Autodesk Fusion 360 part; units mm, degrees
sketch "Sketch1" plane through (0, 0, 0) normal (0, 0, 1) x (1, 0, 0)
  line L0 (-19.8608, 0) -> (46.1392, 0) construction
  line L1 (-17, -9.25) -> (-10, -9.25)
  line L2 (-10, -9.25) -> (-10, -10)
  line L3 (-10, -10) -> (30.5, -10)
  line L4 (30.5, -10) -> (30.5, -9.25)
  line L5 (30.5, -9.25) -> (37.5, -9.25)
  line L6 (37.5, -9.25) -> (37.5, 0)
  circle A0 centre (-13, -4.5) radius 2.25
  line L7 (-17, -9.25) -> (-17, 0)
  circle A1 centre (34.5, -4.5) radius 2.25
  line L8 (30.5, 10) -> (30.5, 9.25)
  line L9 (-10, 9.25) -> (-10, 10)
  line L10 (-17, 9.25) -> (-17, 0)
  line L11 (37.5, 9.25) -> (37.5, 0)
  line L12 (30.5, 9.25) -> (37.5, 9.25)
  circle A2 centre (-13, 4.5) radius 2.25
  line L13 (-10, 10) -> (30.5, 10)
  line L14 (-17, 9.25) -> (-10, 9.25)
  circle A3 centre (34.5, 4.5) radius 2.25
  point P0 (46.1392, 0)
  point P1 (-19.8608, 0)
  dimension "d1" = 4.5
  dimension "d2" = 10
  dimension "d3" = 4.5
  dimension "d4" = 47.5
  dimension "d5" = 7
  dimension "d6" = 7
  dimension "d7" = 4
  dimension "d8" = 4
  dimension "d9" = 4.5
  dimension "d10" = 4.5
  dimension "d11" = 10
  dimension "d12" = 10
  dimension "d13" = 9.25
  dimension "d14" = 9.25
extrude "Extrude1" add sketch "Sketch1" along normal blind 13
sketch "Sketch3" plane through (0, -9.25, 0) normal (0, -1, 0) x (1, 0, 0)
  line L0 (30.5, 0) -> (37.5, 0)
  line L1 (37.5, 0) -> (37.5, 13)
  line L2 (37.5, 13) -> (30.5, 13)
  line L3 (30.5, 13) -> (30.5, 0)
  line L4 (37.5, 0) -> (30.5, 0)
  line L5 (30.5, 0) -> (30.5, 3)
  line L6 (30.5, 3) -> (37.5, 3)
  line L7 (37.5, 3) -> (37.5, 0)
  line L8 (-10, 0) -> (-17, 0)
  line L9 (-17, 0) -> (-17, 3)
  line L10 (-17, 3) -> (-10, 3)
  line L11 (-10, 3) -> (-10, 0)
  dimension "d21" = 3
  dimension "d22" = 3
extrude "Extrude3" cut sketch "Sketch3" against normal blind 26 contours L1 L2 L3 L6
sketch "Sketch4" plane through (0, -9.25, 0) normal (0, -1, 0) x (1, 0, 0)
  line L0 (-17, 0) -> (-10, 0)
  line L1 (-10, 0) -> (-10, 13)
  line L2 (-10, 13) -> (-17, 13)
  line L3 (-17, 13) -> (-17, 0)
  line L4 (-17, 0) -> (-10, 0)
  line L5 (-10, 0) -> (-10, 3)
  line L6 (-10, 3) -> (-17, 3)
  line L7 (-17, 3) -> (-17, 0)
  dimension "d25" = 3
extrude "Extrude4" cut sketch "Sketch4" against normal blind 22 contours L1 L2 L3 L6
sketch "Sketch5" plane through (0, 0, 13) normal (0, 0, 1) x (-1, 0, 0)
  line L0 (10, -10) -> (10, 10)
  line L1 (10, 10) -> (-30.5, 10)
  line L2 (-30.5, 10) -> (-30.5, -10)
  line L3 (-30.5, -10) -> (10, -10)
  circle A0 centre (0, 0) radius 3
  dimension "d28" = 6
extrude "Extrude5" cut sketch "Sketch5" against normal blind 21 contours A0
sketch "Sketch6" plane through (0, 0, 0) normal (0, 0, -1) x (-1, 0, 0)
  circle A0 centre (0, 0) radius 3
  line L0 (10, -10) -> (10, 10)
  line L1 (10, 10) -> (-33, 10)
  line L2 (-33, 10) -> (-33, -10)
  line L3 (-33, -10) -> (10, -10)
  circle A1 centre (-11, 0) radius 0.75
  circle A2 centre (-20.5, 0) radius 0.75
  circle A3 centre (0, 0) radius 3
  circle A4 centre (-34.5, 4.5) radius 2.25
  circle A5 centre (13, -4.5) radius 2.25
  circle A6 centre (-34.5, -4.5) radius 2.25
  circle A7 centre (13, 4.5) radius 2.25
  line L4 (10, -9.25) -> (17, -9.25)
  line L5 (17, -9.25) -> (17, 9.25)
  line L6 (17, 9.25) -> (10, 9.25)
  line L7 (10, 9.25) -> (10, 10)
  line L8 (10, 10) -> (-30.5, 10)
  line L9 (-30.5, 10) -> (-30.5, 9.25)
  line L10 (-30.5, 9.25) -> (-37.5, 9.25)
  line L11 (-37.5, 9.25) -> (-37.5, -9.25)
  line L12 (-37.5, -9.25) -> (-30.5, -9.25)
  line L13 (-30.5, -9.25) -> (-30.5, -10)
  line L14 (-30.5, -10) -> (10, -10)
  line L15 (10, -10) -> (10, -9.25)
  dimension "d31" = 1.5
  dimension "d32" = 1.5
  dimension "d33" = 11
  dimension "d34" = 9.5
extrude "Extrude6" cut sketch "Sketch6" against normal blind 12 contours A1 | A2
sketch "Sketch7" plane through (0, 0, 0) normal (0, 0, -1) x (1, 0, 0)
  circle A0 centre (11, 0) radius 0.75
  circle A1 centre (20.5, 0) radius 0.75
  circle A2 centre (0, 0) radius 3
  circle A3 centre (34.5, -4.5) radius 2.25
  circle A4 centre (-13, 4.5) radius 2.25
  circle A5 centre (34.5, 4.5) radius 2.25
  circle A6 centre (-13, -4.5) radius 2.25
  line L0 (-10, 9.25) -> (-17, 9.25)
  line L1 (-17, 9.25) -> (-17, -9.25)
  line L2 (-17, -9.25) -> (-10, -9.25)
  line L3 (-10, -9.25) -> (-10, -10)
  line L4 (-10, -10) -> (30.5, -10)
  line L5 (30.5, -10) -> (30.5, -9.25)
  line L6 (30.5, -9.25) -> (37.5, -9.25)
  line L7 (37.5, -9.25) -> (37.5, 9.25)
  line L8 (37.5, 9.25) -> (30.5, 9.25)
  line L9 (30.5, 9.25) -> (30.5, 10)
  line L10 (30.5, 10) -> (-10, 10)
  line L11 (-10, 10) -> (-10, 9.25)
  line L12 (29.5, 9) -> (-9, 9)
  line L13 (-9, 9) -> (-9, -9)
  line L14 (-9, -9) -> (29.5, -9)
  line L15 (29.5, -9) -> (29.5, 9)
  line L16 (29.5, 9) -> (-9, -9) construction
  line L17 (-9, 9) -> (29.5, -9) construction
  point P0 (10.25, 0)
  dimension "d37" = 1
  dimension "d38" = 1
  dimension "d39" = 1
  dimension "d40" = 1
extrude "Extrude7" cut sketch "Sketch7" against normal blind 12 contours L12 L13 L14 L15
sketch "Sketch8" plane through (0, 0, 12) normal (0, 0, -1) x (1, 0, 0)
  circle A0 centre (0, 0) radius 3
  line L0 (29.5, -9) -> (29.5, 9)
  line L1 (29.5, 9) -> (-9, 9)
  line L2 (-9, 9) -> (-9, -9)
  line L3 (-9, -9) -> (29.5, -9)
  circle A1 centre (11, 0) radius 0.75
  circle A2 centre (20.5, 0) radius 0.75
  circle A3 centre (11, 0) radius 1.75
  circle A4 centre (20.5, 0) radius 1.75
  dimension "d43" = 1.5
  dimension "d44" = 1.5
  dimension "d45" = 9.5
  dimension "d46" = 11
  dimension "d47" = 3.5
  dimension "d48" = 3.5
extrude "Extrude8" add sketch "Sketch8" along normal blind 1 contours A3 | A4
sketch "Sketch9" plane through (0, 0, 12) normal (0, 0, -1) x (1, 0, 0)
  circle A0 centre (11, 0) radius 1.75
  circle A1 centre (0, 0) radius 3
  line L0 (29.5, -9) -> (29.5, 9)
  line L1 (29.5, 9) -> (-9, 9)
  line L2 (-9, 9) -> (-9, -9)
  line L3 (-9, -9) -> (29.5, -9)
  circle A2 centre (20.5, 0) radius 1.75
  circle A3 centre (0, 0) radius 3
  circle A4 centre (0, 0) radius 5
  dimension "d51" = 2
extrude "Extrude9" add sketch "Sketch9" along normal blind 1 contours A4
sketch "Sketch10" plane through (0, 0, 13) normal (0, 0, 1) x (-1, 0, 0)
  circle A0 centre (0, 0) radius 3
  line L0 (10, -10) -> (10, 10)
  line L1 (10, 10) -> (-30.5, 10)
  line L2 (-30.5, 10) -> (-30.5, -10)
  line L3 (-30.5, -10) -> (10, -10)
  circle A1 centre (0, 0) radius 3
  circle A2 centre (0, 0) radius 5
  dimension "d54" = 2
extrude "Extrude10" add sketch "Sketch10" along normal blind 2 contours A2
fillet "Fillet1" radius 1 4 edges at (30.5, -10, 6.5) (30.5, 10, 6.5) (-10, -10, 6.5) (-10, 10, 6.5)
fillet "Fillet2" radius 2 4 edges at (37.5, -9.25, 1.5) (37.5, 9.25, 1.5) (-17, -9.25, 1.5) (-17, 9.25, 1.5)
sketch "Sketch11" plane through (0, 0, 12) normal (0, 0, -1) x (1, 0, 0)
  circle A0 centre (0, 0) radius 5 construction
  circle A1 centre (11, 0) radius 1.75 construction
  line L0 (29.5, -9) -> (29.5, 9) construction
  line L1 (29.5, 9) -> (-9, 9) construction
  line L2 (-9, 9) -> (-9, -9) construction
  line L3 (-9, -9) -> (29.5, -9) construction
  circle A2 centre (20.5, 0) radius 1.75 construction
  line L4 (28.25, -7.5) -> (-7.75, -7.5) construction
  line L5 (-7.75, -7.5) -> (-7.75, 7.5) construction
  line L6 (-7.75, 7.5) -> (28.25, 7.5) construction
  line L7 (28.25, 7.5) -> (28.25, -7.5) construction
  circle A3 centre (-7.75, 7.5) radius 0.875
  circle A4 centre (-7.75, -7.5) radius 0.875
  circle A5 centre (28.25, 7.5) radius 0.875
  circle A6 centre (28.25, -7.5) radius 0.875
  circle A7 centre (28.25, 7.5) radius 1.875
  circle A8 centre (28.25, -7.5) radius 1.875
  circle A9 centre (-7.75, -7.5) radius 1.875
  circle A10 centre (-7.75, 7.5) radius 1.875
  line L8 (-9, 10) -> (29.5, 10)
  line L9 (-9, -10) -> (29.5, -10)
  dimension "d63" = 1.25
  dimension "d66" = 1.75
  dimension "d67" = 1
  dimension "d70" = 36
  dimension "d71" = 15
  dimension "d73" = 2.5
  dimension "d74" = 2.5
  dimension "d75" = 1.25
  dimension "d76" = 1.25
extrude "Extrude11" add sketch "Sketch11" along normal blind 12
equation "d13 = ( 18.5 / 2 ) * 1 mm"
equation "d14 = ( 18.5 / 2 ) * 1 mm"
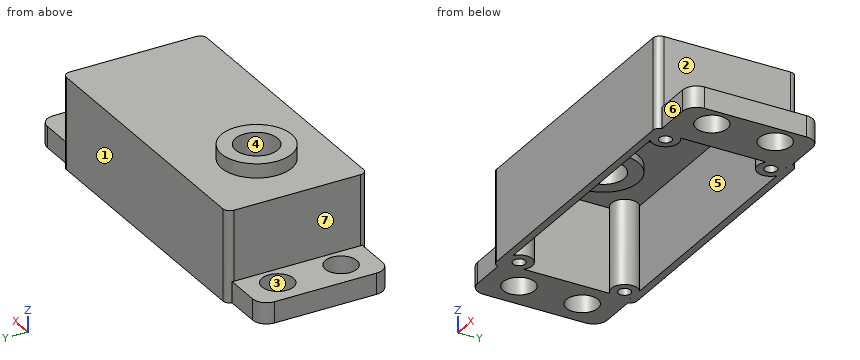
Here's how the part is built. I have some questions about the finished solid (model axes, mm). Face numbers are marked on the shaded views. A direction names the side the tool comes from. Round coordinates to 2 decimals unless told otherwise and drop trailing zeros. Order: outer loops, then holes, each group sorted by start corner. A loop starts at its lowest first (then second) coordinate and runs counter-clockwise, first axis right, second up. Notation, with made-up numbers: (45.5, 79) -> (75.5, 79) arc R17 cw to (75.5, 93) -> close; hole circle Ø11 at (6.5, -16). An arc over 180 degrees is marked (long way). Use CSV: the item, a comma, the result in double quotes.
1. Which directions (+Z, -Z, +X, -X, +Y, -Y) give clear straight access to the entire face, cutting with the end or side of a thin tool? Please do the marked faces 5, 6 and 7.
Recorded:
face 5,"-Z"
face 6,"+Z, -Z, +X, -Y"
face 7,"+Z, -X, +Y, -Y"
2. I want a section at A-A on x = 0. List the corners of the cut face in (y, z) for me, and give its area (3 significant figures).
Recorded:
outline,"(-10, 0) -> (-9, 0) -> (-9, 12) -> (-5, 12) -> (-5, 11) -> (-3, 11) -> (-3, 15) -> (-5, 15) -> (-5, 13) -> (-10, 13) -> close; (3, 11) -> (5, 11) -> (5, 12) -> (9, 12) -> (9, 0) -> (10, 0) -> (10, 13) -> (5, 13) -> (5, 15) -> (3, 15) -> close"
area,"50.0 mm2"
3. I need wall thicknesses on line 1 along X through (y, z) = (-7.5, 7.25) (3 decimals); line 2 along X through (y, z) = (-4.5, 1.05); line 3 along Y through (x, z) = (3.5, 1.75). Which ranges of each line are inside material? Lowest first, please.
Recorded:
line 1,"x = -10 to -8.625, -6.875 to -5.875, 26.375 to 27.375, 29.125 to 30.5"
line 2,"x = -17 to -15.25, -10.75 to -9, 29.5 to 32.25, 36.75 to 37.5"
line 3,"y = -10 to -9, 9 to 10"
4. I want a section at B-B on z = 4.5. Give the number of separate pieces and of enclosed holes in the cut face, and give its area (3 significant figures).
Recorded:
separate pieces,"1"
enclosed holes,"9"
area,"144 mm2"
5. I'm going to push flat-ended pins straight in: P1, Ø4, axis at x = 11, y = 0.5, coming from the -Z side; P2, Ø2.5, axis at x = 34, z = 1, coming from the -Y side; P3, Ø4, axis at y = 6.5, z = 13.5, coming from the +X side. Where does each tip first touch, or does it pass through?
Recorded:
P1,"stops at z = 11"
P2,"stops at y = -9.25"
P3,"stops at x = 30.5"
6. Thinking about a two-plate mould opening in X: for the marked faces 1, 2, 3 and 4, which applies, pulls with the +X half, pulls with the -X half, needs draft (parallel to the pull), parting line crosses it, or undercut?
Recorded:
face 1,"needs draft"
face 2,"pulls with the +X half"
face 3,"undercut"
face 4,"undercut"
7. I want a section at D-D on y = 4.5. List the corners of the cut face in (x, z) for me.
Recorded:
outline,"(-17, 0) -> (-15.25, 0) -> (-15.25, 3) -> (-17, 3) -> close; (-10.75, 0) -> (-9, 0) -> (-9, 12) -> (-2.18, 12) -> (-2.18, 11) -> (2.18, 11) -> (2.18, 12) -> (29.5, 12) -> (29.5, 0) -> (32.25, 0) -> (32.25, 3) -> (30.5, 3) -> (30.5, 13) -> (2.18, 13) -> (2.18, 15) -> (-2.18, 15) -> (-2.18, 13) -> (-10, 13) -> (-10, 3) -> (-10.75, 3) -> close; (36.75, 0) -> (37.5, 0) -> (37.5, 3) -> (36.75, 3) -> close"
